For this review, use the dimensioned drawing (mm, ordinates from the lowest corner) and the shaded views. A direction names the side the tool comes from. Round coordinates to 2 decimals unless told otherwise and drop trailing zeros. Write each loop counter-clockwise with the first axis right and the second up, starting at its lowest first coordinate (ties: lowest second). Pieces come first, ordered by that corner, then holes. Notation, with made-up numbers: M 51,-39.75 L 97,-39.75 A17 ccw 97,-11.75 Z; hole C -3,2.5 d10. An arc over 180 degrees is marked long. Write each question's results on one line, items separated by ' | '. Start each with the question number.
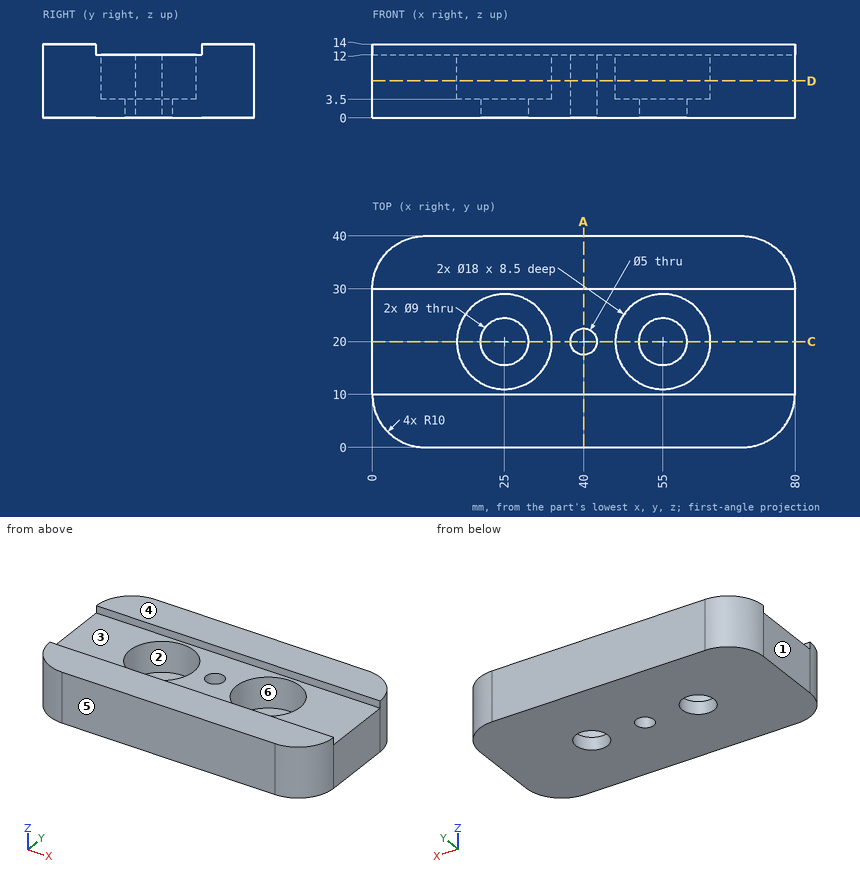
Item 1: For the marked faces 1 and 2, list the 3-axis set-ups (+Z, -Z, +X, -X, +Y, -Y) from which the entire face can be reached by the end or side of a thin tool; tool diameter is ignored.
Item 2: Insertion check: P1, Ø7, axis at x = 55, y = 20, coming from the -Z side; P2, Ø5.5, axis at x = 27, y = 19, coming from the +Z side; P3, Ø4, axis at y = 9, z = 6.5, coming from the +X side. Each pin has a flat end and moves straight along its axis. Give the tip position at first contact, or say it passes through.
Item 3: We need section D-D on z = 7. State the section outline as (x, y) points, then the cut area to 3 significant figures.
Item 4: Mouldability with a two-part tool opening along Y and no side actions: class the marked faces 3, 4, 5 and 6 as pulls with the +Y half, pulls with the -Y half, needs draft (parallel to the pull), parting line crosses it, or undercut.
Item 5: We need section A-A on x = 40. State the section outline as (y, z) points.
Item 6: We need section C-C on y = 20. State the section outline as (x, z) points, then the cut area to 3 significant figures.
Item 7: For probe 1 along X at (y, z) = (18, 4.5) (1 decimal); probe 2 along X at (y, z) = (14, 7.5); probe 3 along Y at (x, z) = (50.5, 13.25), list the stretches that pass through material, from the lowest coordinate up.
Numbers:
1) face 1: +Z, -Z, -X, +Y, -Y | face 2: +Z
2) P1: passes through | P2: stops at z = 3.5 | P3: stops at x = 80
3) outline: M 0,10 A10 ccw 10,0 L 70,0 A10 ccw 80,10 L 80,30 A10 ccw 70,40 L 10,40 A10 ccw 0,30 Z; hole C 25,20 d18; hole C 40,20 d5; hole C 55,20 d18 | area: 2,590 mm^2
4) face 3: undercut | face 4: needs draft | face 5: pulls with the -Y half | face 6: undercut
5) outline: M 0,0 L 17.5,0 L 17.5,12 L 10,12 L 10,14 L 0,14 Z; M 22.5,0 L 40,0 L 40,14 L 30,14 L 30,12 L 22.5,12 Z
6) outline: M 0,0 L 20.5,0 L 20.5,3.5 L 16,3.5 L 16,12 L 0,12 Z; M 29.5,0 L 37.5,0 L 37.5,12 L 34,12 L 34,3.5 L 29.5,3.5 Z; M 42.5,0 L 50.5,0 L 50.5,3.5 L 46,3.5 L 46,12 L 42.5,12 Z; M 59.5,0 L 80,0 L 80,12 L 64,12 L 64,3.5 L 59.5,3.5 Z | area: 531 mm^2
7) probe 1: x = 0 to 16.2, 33.8 to 38.5, 41.5 to 46.2, 63.8 to 80 | probe 2: x = 0 to 18.29, 31.71 to 48.29, 61.71 to 80 | probe 3: y = 0 to 10, 30 to 40
